For this review, use the dimensioned drawing (mm, ordinates from the lowest corner) and the shaded views. A direction names the side the tool comes from. Coordinates: 2 decimals unless noted, no trailing zeros. Write each loop counter-clockwise with the first axis right and the second up, starting at its lowest first coordinate (ties: lowest second). Pieces come first, ordered by that corner, then holes.
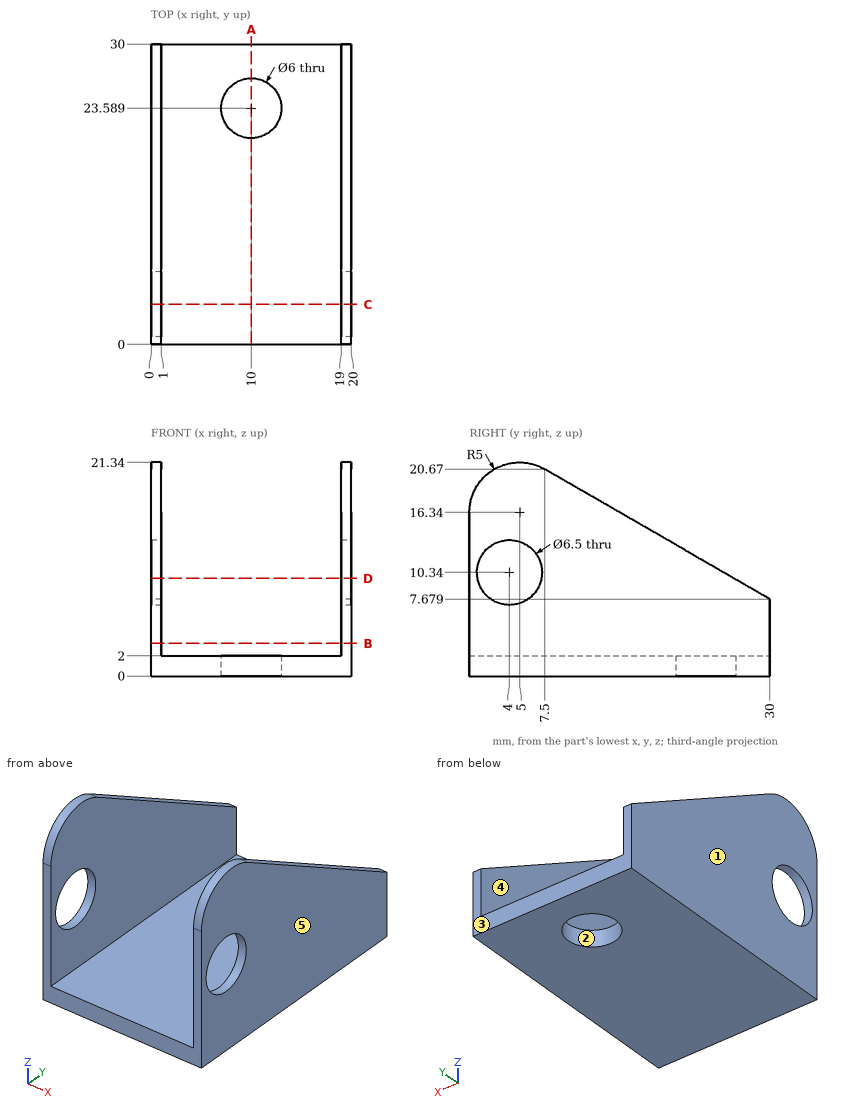
Item 1: Take a section at A-A, the plane x = 10. Write out the cut boundary in (y, z).
Solved:
outline: (0, 0) - (20.59, 0) - (20.59, 2) - (0, 2) - close; (26.59, 0) - (30, 0) - (30, 2) - (26.59, 2) - close
Item 2: Mouldability with a two-part tool opening along Y and no side actions: class the marked faces 1, 2 and 3 as pulls with the +Y half, pulls with the -Y half, needs draft (parallel to the pull), parting line crosses it, or undercut.
Solved:
face 1: needs draft
face 2: undercut
face 3: pulls with the +Y half
Item 3: Take a section at B-B, the plane z = 3.25. Write out the cut boundary in (x, y).
Solved:
outline: (0, 0) - (1, 0) - (1, 30) - (0, 30) - close; (19, 0) - (20, 0) - (20, 30) - (19, 30) - close
Item 4: To check wall thickness, follow line 1 along X through (y, z) = (25.5, 9.25); line 2 along Z through (x, y) = (10, 8). State the ranges of each line that lie inside material, in increasing order.
Solved:
line 1: x = 0 to 1, 19 to 20
line 2: z = 0 to 2
Item 5: Machinability: for the marked faces 4 and 5, which of the approach directions +Z, -Z, +X, -X, +Y, -Y give a long, thin tool a straight path to every point of the face, cutting with its end or side? Answer none if there is none.
Solved:
face 4: +Z, +Y, -Y
face 5: +Z, -Z, +X, +Y, -Y
Item 6: Take a section at D-D, the plane z = 9.75. Write out the cut boundary in (x, y).
Solved:
outline: (0, 0) - (1, 0) - (1, 0.8) - (0, 0.8) - close; (0, 7.2) - (1, 7.2) - (1, 26.41) - (0, 26.41) - close; (19, 0) - (20, 0) - (20, 0.8) - (19, 0.8) - close; (19, 7.2) - (20, 7.2) - (20, 26.41) - (19, 26.41) - close
Item 7: Take a section at C-C, the plane y = 4. Write out the cut boundary in (x, z).
Solved:
outline: (0, 0) - (20, 0) - (20, 7.09) - (19, 7.09) - (19, 2) - (1, 2) - (1, 7.09) - (0, 7.09) - close; (0, 13.59) - (1, 13.59) - (1, 21.24) - (0, 21.24) - close; (19, 13.59) - (20, 13.59) - (20, 21.24) - (19, 21.24) - close
Item 8: For pin 1 (8 mm diameter, centred on x = 9.5, y = 16, fed in from +Z), flat-tipped, find the tip position at first contact; note if it passes through.
Solved:
pin 1: stops at z = 2
